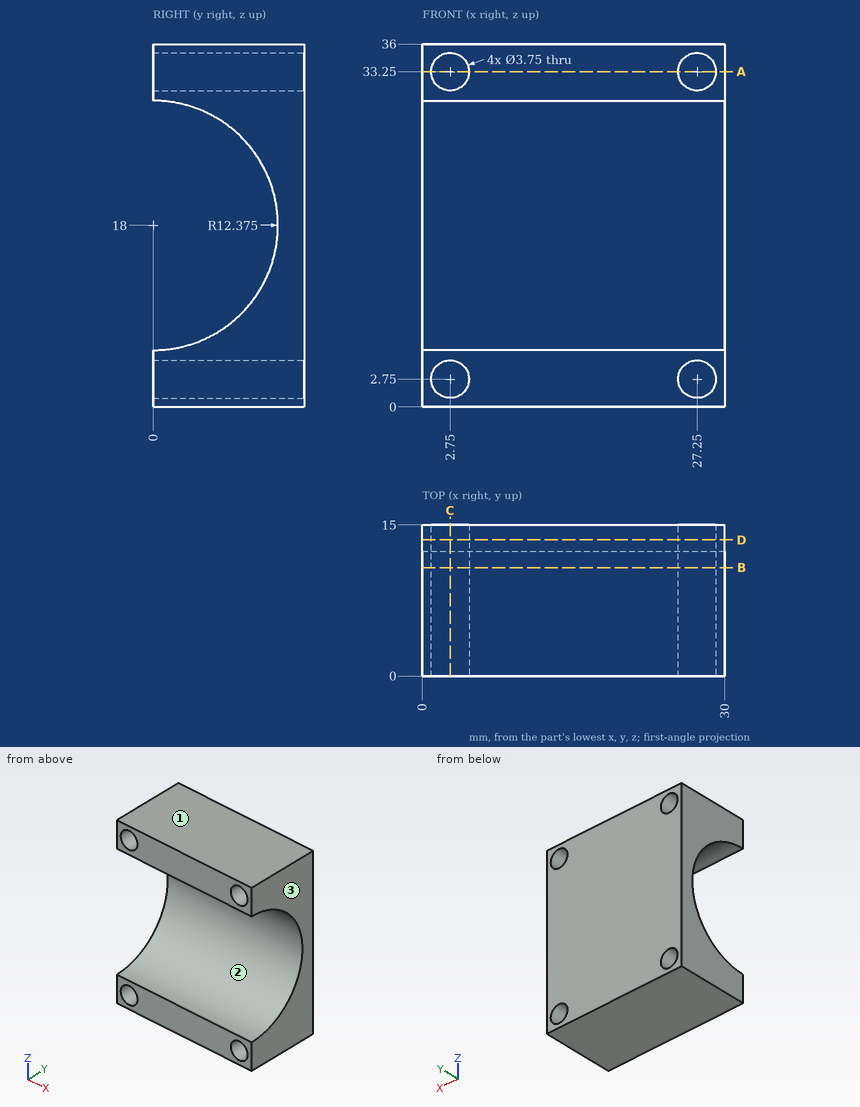
Design review of the part shown in the three views and the two pictorial views. Dimensions are in mm from the part's minimum x, y and z. Give positions to 0.01 mm unless a question says otherwise; leave off trailing zeros. Order: outer loops, then holes, each group sorted by start corner. A loop starts at its lowest first (then second) coordinate and runs counter-clockwise, first axis right, second up. Notation, with made-up numbers: M 88.25,-37 L 110.25,-37 A26 cw 110.25,-5 Z; hole C 12.25,41.25 d10. An arc over 180 degrees is marked long. Answer in a Markdown table with one row per item. Add a question column.
(1) Consider section A-A on z = 33.25. State the section outline as (x, y) points (3 decimals), and give its area (4 significant figures).
(2) Consider section D-D on y = 13.5. State the section outline as (x, z) points (3 decimals), and give its area (3 significant figures).
(3) Consider section C-C on x = 2.75. State the section outline as (y, z) points (3 decimals), and give its area (3 significant figures).
(4) Consider section B-B on y = 10.75. State the section outline as (x, z) points (3 decimals).
(5) For pin 1 (5 mm diameter, centred on x = 4.5, z = 14, fed in from -Y); pin 2 (5 mm diameter, centred on x = 19, z = 18.5, fed in from -Y); pin 3 (2 mm diameter, centred on x = 27.25, z = 33.25, fed in from +Y), all flat-tipped, find the tip position at first contact; note any pin that passes through.
(6) Mouldability with a two-part tool opening along Z and no side actions: class the marked faces 1, 2 and 3 as +Z half, -Z half, draft (parallel to the pull), parting line (faces both ways), or undercut.
(7) Wall thickness on probe 1 along X at (y, z) = (11.75, 2.75) (3 decimals); probe 2 along Z at (x, y) = (2.75, 3.25) (3 decimals); probe 3 along X at (y, z) = (7, 4): over which ranges is each line inside the solid? List them lowest first. Write a range as [from, to].
Evaluation:
| question | item | result |
|---|---|---|
| 1 | outline | M 0,0 L 0.875,0 L 0.875,15 L 0,15 Z; M 4.625,0 L 25.375,0 L 25.375,15 L 4.625,15 Z; M 29.125,0 L 30,0 L 30,15 L 29.125,15 Z |
| 1 | area | 337.5 mm^2 |
| 2 | outline | M 0,0 L 30,0 L 30,36 L 0,36 Z; hole C 2.75,2.75 d3.75; hole C 2.75,33.25 d3.75; hole C 27.25,2.75 d3.75; hole C 27.25,33.25 d3.75 |
| 2 | area | 1,040 mm^2 |
| 3 | outline | M 0,0 L 15,0 L 15,0.875 L 0,0.875 Z; M 0,4.625 L 15,4.625 L 15,31.375 L 0,31.375 L 0,30.375 A12.375 cw 0,5.625 Z; M 0,35.125 L 15,35.125 L 15,36 L 0,36 Z |
| 3 | area | 187 mm^2 |
| 4 | outline | M 0,0 L 30,0 L 30,11.87 L 0,11.87 Z; M 0,24.13 L 30,24.13 L 30,36 L 0,36 Z; hole C 2.75,2.75 d3.75; hole C 2.75,33.25 d3.75; hole C 27.25,2.75 d3.75; hole C 27.25,33.25 d3.75 |
| 5 | pin 1 | stops at y = 10.53 |
| 5 | pin 2 | stops at y = 12.01 |
| 5 | pin 3 | passes through |
| 6 | face 1 | +Z half |
| 6 | face 2 | undercut |
| 6 | face 3 | draft |
| 7 | probe 1 | x = [0, 0.875], [4.625, 25.375], [29.125, 30] |
| 7 | probe 2 | z = [0, 0.875], [4.625, 6.059], [29.941, 31.375], [35.125, 36] |
| 7 | probe 3 | x = [0, 1.35], [4.15, 25.85], [28.65, 30] |
